from build123d import *

# Parameters (mm, degrees)
SKETCH1_W           = 61
SKETCH1_H           = 61
BOSS_EXTRUDE1_DEPTH = 3
SKETCH2_W           = 3
SKETCH2_H           = 8
SKETCH2_H_2         = 7
SKETCH2_W_2         = 8
SKETCH2_H_3         = 3
SKETCH2_W_3         = 7
CUT_EXTRUDE1_DEPTH  = 3
CUT_EXTRUDE2_DEPTH  = 3


with BuildPart() as part:
    # Sketch1 → Boss-Extrude1 (new body)
    with BuildSketch(Plane.XY):
        Rectangle(SKETCH1_W, SKETCH1_H)
    extrude(amount=BOSS_EXTRUDE1_DEPTH)

    # Sketch2 → Cut-Extrude1 (cut)
    with BuildSketch(Plane.XY.offset(3)):
        with Locations((-29, 15.5)):
            Rectangle(SKETCH2_W, SKETCH2_H)
        with Locations((-29, 0)):
            Rectangle(SKETCH2_W, SKETCH2_H_2)
        with Locations((-29, -15.5)):
            Rectangle(SKETCH2_W, SKETCH2_H)
        with Locations((-15.5, -29)):
            Rectangle(SKETCH2_W_2, SKETCH2_H_3)
        with Locations((0, -29)):
            Rectangle(SKETCH2_W_3, SKETCH2_H_3)
        with Locations((15.5, -29)):
            Rectangle(SKETCH2_W_2, SKETCH2_H_3)
        with Locations((29, -15.5)):
            Rectangle(SKETCH2_W, SKETCH2_H)
        with Locations((29, 0)):
            Rectangle(SKETCH2_W, SKETCH2_H_2)
        with Locations((29, 15.5)):
            Rectangle(SKETCH2_W, SKETCH2_H)
        with Locations((15.5, 29)):
            Rectangle(SKETCH2_W_2, SKETCH2_H_3)
        with Locations((0, 29)):
            Rectangle(SKETCH2_W_3, SKETCH2_H_3)
        with Locations((-15.5, 29)):
            Rectangle(SKETCH2_W_2, SKETCH2_H_3)
    extrude(amount=-CUT_EXTRUDE1_DEPTH, mode=Mode.SUBTRACT)

    # Sketch3 → Cut-Extrude2 (cut)
    with BuildSketch(Plane.XY.offset(3)):
        with BuildLine():
            ThreePointArc((-12.5, 11), (-15.060660172, 12.060660172), (-14, 9.5))
            Line((-14, 9.5), (-14, 11))
            Line((-14, 11), (-12.5, 11))
        make_face()
        with BuildLine():
            Line((-14, 11), (-14, 9.5))
            ThreePointArc((-14, 9.5), (-12.939339828, 9.939339828), (-12.5, 11))
            Line((-12.5, 11), (-14, 11))
        make_face()
        with BuildLine():
            ThreePointArc((12.5, 11), (12.939339828, 9.939339828), (14, 9.5))
            Line((14, 9.5), (14, 11))
            Line((14, 11), (12.5, 11))
        make_face()
        with BuildLine():
            Line((14, 11), (14, 9.5))
            ThreePointArc((14, 9.5), (15.060660172, 9.939339828), (15.5, 11))
            ThreePointArc((15.5, 11), (14, 12.5), (12.5, 11))
            Line((12.5, 11), (14, 11))
        make_face()
        with BuildLine():
            Line((-14, -9.5), (-14, -11))
            Line((-14, -11), (-12.5, -11))
            ThreePointArc((-12.5, -11), (-12.939339828, -9.939339828), (-14, -9.5))
        make_face()
        with BuildLine():
            Line((-12.5, -11), (-14, -11))
            Line((-14, -11), (-14, -9.5))
            ThreePointArc((-14, -9.5), (-15.060660172, -12.060660172), (-12.5, -11))
        make_face()
        with BuildLine():
            ThreePointArc((14, -9.5), (12.939339828, -9.939339828), (12.5, -11))
            Line((12.5, -11), (14, -11))
            Line((14, -11), (14, -9.5))
        make_face()
        with BuildLine():
            Line((14, -11), (12.5, -11))
            ThreePointArc((12.5, -11), (14, -12.5), (15.5, -11))
            ThreePointArc((15.5, -11), (15.060660172, -9.939339828), (14, -9.5))
            Line((14, -9.5), (14, -11))
        make_face()
    extrude(amount=-CUT_EXTRUDE2_DEPTH, mode=Mode.SUBTRACT)


solid = part.part
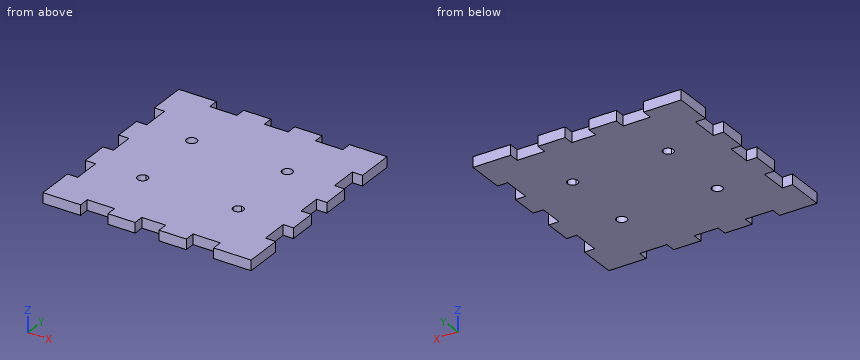
The model under review builds one solid part; all positions refer to its coordinate system, in mm. Give positions to 0.01 mm unless a question says otherwise; leave off trailing zeros. Order: outer loops, then holes, each group sorted by start corner. A loop starts at its lowest first (then second) coordinate and runs counter-clockwise, first axis right, second up. Notation, with made-up numbers: M 83.25,-20.75 L 136.25,-20.75 A14 ccw 136.25,-2.75 Z; hole C -36,-0.5 d11. An arc over 180 degrees is marked long. Answer in a Markdown table with one row per item. Add a question column.
1. Add section B-B on x = -1. State the section outline as (y, z) points, plus the area to 3 significant figures.
2. Add section A-A on z = 2.3. Count the separate pieces of the cut face and the enclosed holes in it, plus the area to 3 significant figures.
3. To check wall thickness, follow line 1 along X through (y, z) = (11, 1.3); line 2 along Y through (x, z) = (-14, 2.2); line 3 along X through (y, z) = (-3, 1.25). State the ranges of each line that lie inside material, in increasing order.
4. For pin 1 Ø1.5 at (x, z) = (-16, 1.5) entering from +Y, flat-tipped, find the tip position at first contact; note if it passes through.
The answers:
| question | item | result |
|---|---|---|
| 1 | outline | M -27.5,0 L 27.5,0 L 27.5,3 L -27.5,3 Z |
| 1 | area | 165 mm2 |
| 2 | separate pieces | 1 |
| 2 | enclosed holes | 4 |
| 2 | area | 3,420 mm2 |
| 3 | line 1 | -30.5 to -15.5, -12.5 to 12.5, 15.5 to 30.5 |
| 3 | line 2 | -27.5 to -12.5, -9.5 to 9.5, 12.5 to 27.5 |
| 3 | line 3 | -27.5 to 27.5 |
| 4 | pin 1 | y = 27.5 |
